Verification items for this drawing (mm, ordinates from the low corner). Round coordinates to 2 decimals unless told otherwise and drop trailing zeros. Loops run counter-clockwise (first coordinate to the right, second up) from the corner with the lowest first, then second, coordinate; pieces in that order, holes last. Notation, with made-up numbers: (5, -25) -> (11, -25) arc R16 cw to (11, -19) -> close; hole circle Ø9 at (-16, 20.25). An arc over 180 degrees is marked (long way). One line per item, written item: value. Start each with the question number.
1. Cross-section at B-B on x = 214.63. Record the cut outline in (y, z), then the cut area to 3 significant figures.
2. Go/stop test with flat-tipped pins: pin 1 (8 mm diameter, centred on y = 3, z = 77, fed in from -X); pin 2 (5.5 mm diameter, centred on x = 214.63, z = 63.5, fed in from +Y). Record where each tip stops, or that it passes through.
3. Cross-section at A-A on z = 63.5. Record the cut outline in (x, y).
4. Material ranges on L1, parallel to Z at x = 177.8, y = 13.5; L2, parallel to X at y = 15.25, z = 60.5, recorded low to high.
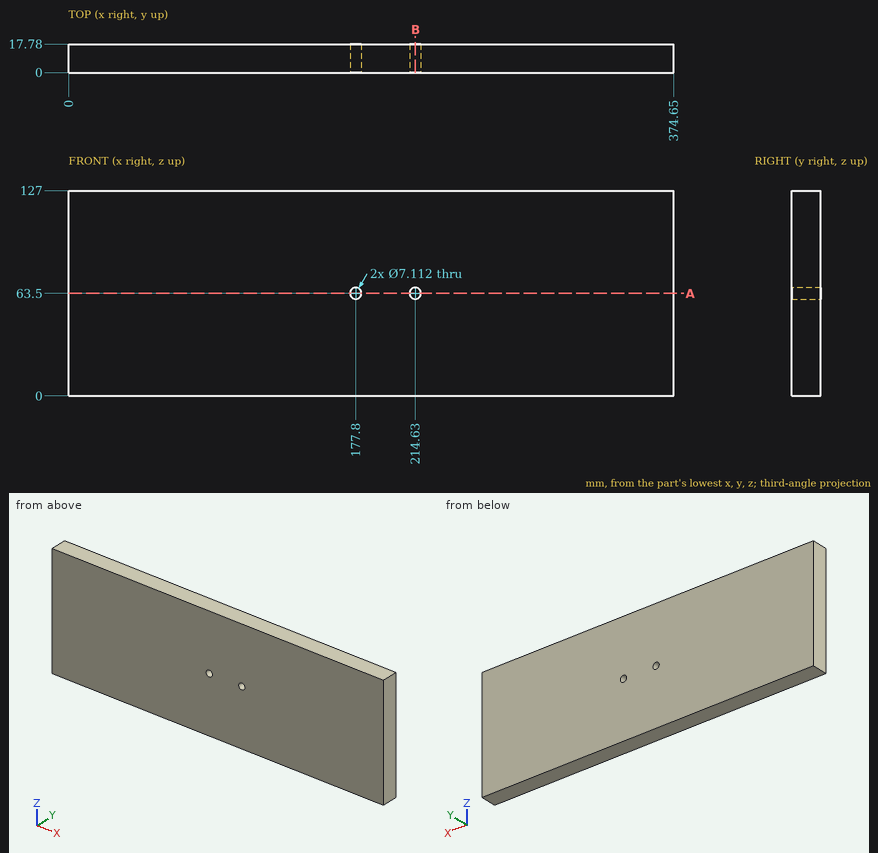
Taken from the geometry:
1. outline: (0, 0) -> (17.78, 0) -> (17.78, 59.94) -> (0, 59.94) -> close; (0, 67.06) -> (17.78, 67.06) -> (17.78, 127) -> (0, 127) -> close
1. area: 2,130 mm2
2. pin 1: stops at x = 0
2. pin 2: passes through
3. outline: (0, 0) -> (174.24, 0) -> (174.24, 17.78) -> (0, 17.78) -> close; (181.36, 0) -> (211.07, 0) -> (211.07, 17.78) -> (181.36, 17.78) -> close; (218.19, 0) -> (374.65, 0) -> (374.65, 17.78) -> (218.19, 17.78) -> close
4. L1: z = 0 to 59.94, 67.06 to 127
4. L2: x = 0 to 175.89, 179.71 to 212.72, 216.54 to 374.65
